The listing builds one solid part. Answer for the finished solid, in the listing's coordinates (mm). A direction names the side the tool comes from. Round coordinates to 2 decimals unless told otherwise and drop trailing zeros. Write each loop counter-clockwise with the first axis right and the second up, starting at its lowest first coordinate (ties: lowest second). Pieces come first, ordered by that corner, then holes. Notation, with made-up numbers: (-23, -3) - (12, -3) arc R22 ccw to (12, 25) - close; hole circle Ø10 at (53.5, 14). An arc over 180 degrees is marked (long way). Return JSON: item names as keys, results as strings. Group by question number.
(1) Section D-D, the plane y = -7 is taken. Write down the section's boundary in (x, z).
(2) Determine the mould class of faces 1 (the flat face through (1.928, -5, 1)), 2 (the flat face through (0, -4, 1)), 3 (the flat face through (1, -8.28, 1)) for opening direction Y: +Y half, -Y half, draft (parallel to the pull), parting line (faces both ways), or undercut.
(3) Which of the six approach directions +Z, -Z, +X, -X, +Y, -Y give full straight-line access (tool end or side, diameter ignored) to faces 4 (the cylindrical face through (1.161, -7.434, 1.166)), 5 (the flat face through (1, 0, 1))?
(4) Find the intervals of material crossed by line 1 along X through (y, z) = (-5.25, 0.7); line 2 along Y through (x, z) = (1.3, 1.5); line 3 along Y through (x, z) = (1.4, 1.7), in increasing order. Write a range as [from, to].
(5) This flat-tipped pin is pushed along its axis until it touches: pin 1 (1 mm diameter, centred on x = 0, y = -6.5, fed in from -Z). Where does it stop, or does it pass through?
(6) Section A-A, the plane y = -5.75 is taken. Write down the section's boundary in (x, z), then the cut area to 3 significant figures.
(7) Section B-B, the plane z = 0.3 is taken. Give the number of separate pieces and of enclosed holes in the cut face, then the cut area to 3 significant figures.
```python
from build123d import *

# Parameters (mm, degrees)
SKETCH1_W           = 2.3
SKETCH1_H           = 8.28
BOSS_EXTRUDE1_DEPTH = 2.3
SKETCH4_R           = 0.75
CUT_EXTRUDE3_DEPTH  = 2.627407371
FILLET7_R           = 0.2
FILLET8_R           = 0.2
FILLET9_R           = 0.2
FILLET10_R          = 0.2
FILLET12_R          = 0.15
FILLET13_R          = 0.15
SKETCH9_R           = 0.747027578
SKETCH9_R_2         = 0.752905599
SKETCH9_W           = 1.5
SKETCH9_H           = 3.5
CUT_EXTRUDE4_DEPTH  = 2.3


with BuildPart() as part:
    # Sketch1 → Boss-Extrude1 (new body)
    with BuildSketch(Plane.XY):
        with Locations((1.15, -4.14)):
            Rectangle(SKETCH1_W, SKETCH1_H)
    extrude(amount=BOSS_EXTRUDE1_DEPTH)

    # Sketch4 → Cut-Extrude3 (cut)
    with BuildSketch(Plane(origin=(-0.047615046, -0.231066523, 2.3), x_dir=(1, 0, 0), z_dir=(0, 0, 1))):
        with Locations((1.200582347, -0.913587841)):
            Circle(SKETCH4_R)
    extrude(amount=-CUT_EXTRUDE3_DEPTH, mode=Mode.SUBTRACT)

    # Fillet7
    fillet7_edges = [part.edges().sort_by_distance(p)[0] for p in [
        (1.15, 0, 2.3),
    ]]
    fillet(fillet7_edges, radius=FILLET7_R)

    # Fillet8
    fillet8_edges = [part.edges().sort_by_distance(p)[0] for p in [
        (2.3, -4.24, 2.3),
        (2.3, 0, 1.05),
        (2.3, -0.058578644, 2.241421356),
    ]]
    fillet(fillet8_edges, radius=FILLET8_R)

    # Fillet9
    fillet9_edges = [part.edges().sort_by_distance(p)[0] for p in [
        (0, -4.24, 2.3),
        (0, 0, 1.05),
        (0, -0.058578644, 2.241421356),
    ]]
    fillet(fillet9_edges, radius=FILLET9_R)

    # Fillet10
    fillet10_edges = [part.edges().sort_by_distance(p)[0] for p in [
        (2.3, -8.28, 1.05),
        (2.241421356, -8.28, 2.241421356),
        (0, -8.28, 1.05),
        (1.15, -8.28, 2.3),
        (0.058578644, -8.28, 2.241421356),
    ]]
    fillet(fillet10_edges, radius=FILLET10_R)

    # Fillet12
    fillet12_edges = [part.edges().sort_by_distance(p)[0] for p in [
        (0.402967301, -1.144654364, 2.3),
    ]]
    fillet(fillet12_edges, radius=FILLET12_R)

    # Fillet13
    fillet13_edges = [part.edges().sort_by_distance(p)[0] for p in [
        (0.402967301, -1.144654364, 0),
    ]]
    fillet(fillet13_edges, radius=FILLET13_R)

    # Sketch9 → Cut-Extrude4 (cut)
    with BuildSketch(Plane(origin=(0, -0.220326659, 2.3), x_dir=(1, 0, 0), z_dir=(0, 0, 1))):
        with Locations((1.178039953, -2.960502764)):
            Circle(SKETCH9_R)
        with Locations((1.178039953, -6.460502764)):
            Circle(SKETCH9_R_2)
        with Locations((1.178039953, -4.710502764)):
            Rectangle(SKETCH9_W, SKETCH9_H)
    extrude(amount=-CUT_EXTRUDE4_DEPTH, mode=Mode.SUBTRACT)


solid = part.part
```
Working result:
{
 "1": {"outline": "(0, 0) - (0.5, 0) - (0.5, 2.3) - (0.2, 2.3) arc R0.2 ccw to (0, 2.1) - close; (1.86, 0) - (2.3, 0) - (2.3, 2.1) arc R0.2 ccw to (2.1, 2.3) - (1.86, 2.3) - close"},
 "2": {"face 1": "undercut", "face 2": "draft", "face 3": "-Y half"},
 "3": {"face 4": "+Z, -Z", "face 5": "+Z, -Z, +X, -X, +Y"},
 "4": {"line 1": "x = [0, 0.43], [1.93, 2.3]", "line 2": "y = [-8.28, -7.42], [-2.44, -1.88], [-0.41, 0]", "line 3": "y = [-8.28, -7.4], [-2.47, -1.85], [-0.44, 0]"},
 "5": {"pin 1": "stops at z = 0"},
 "6": {"outline": "(0, 0) - (0.43, 0) - (0.43, 2.3) - (0.2, 2.3) arc R0.2 ccw to (0, 2.1) - close; (1.93, 0) - (2.3, 0) - (2.3, 2.1) arc R0.2 ccw to (2.1, 2.3) - (1.93, 2.3) - close", "area": "1.82 mm^2"},
 "7": {"separate pieces": "1", "enclosed holes": "2", "area": "10.2 mm^2"}
}
